Drawing for the job (mm, zero at the part's lowest x, y, z). Round coordinates to 2 decimals unless told otherwise and drop trailing zeros. Write each loop counter-clockwise with the first axis right and the second up, starting at its lowest first coordinate (ties: lowest second). Pieces come first, ordered by that corner, then holes. Notation, with made-up numbers: M -16,-29.75 L 10,-29.75 A25 ccw 10,-0.75 Z; hole C 20,42 d8. An arc over 180 degrees is marked long. Use a Markdown table: item, result. Add a question column.
1) Slice it at A-A on z = 27.5. Write the cut outline in (x, y).
2) Wall check: probe 1 along Z at (x, y) = (66.04, 2.55); probe 2 along Z at (x, y) = (61.5, 1.55); probe 3 along X at (y, z) = (1.4, 19). Give the ranges that are in metal, low to high.
3) Slice it at D-D on x = 66.04. Write the cut outline in (y, z).
4) Drop flat-ended pins along their axis: P1, Ø1.1, axis at y = 2, z = 50, coming from the -X side; P2, Ø1.1, axis at y = 3, z = 8.5, coming from the +X side; P3, Ø0.8, axis at x = 106, y = 1, coming from the -Z side. Give the stop position or say it passes through.
5) Slice it at C-C on x = 54. Write the cut outline in (y, z).
6) Slice it at B-B on y = 2.95. Give the number of separate pieces and of enclosed holes in the cut face, plus the area to 3 significant figures.
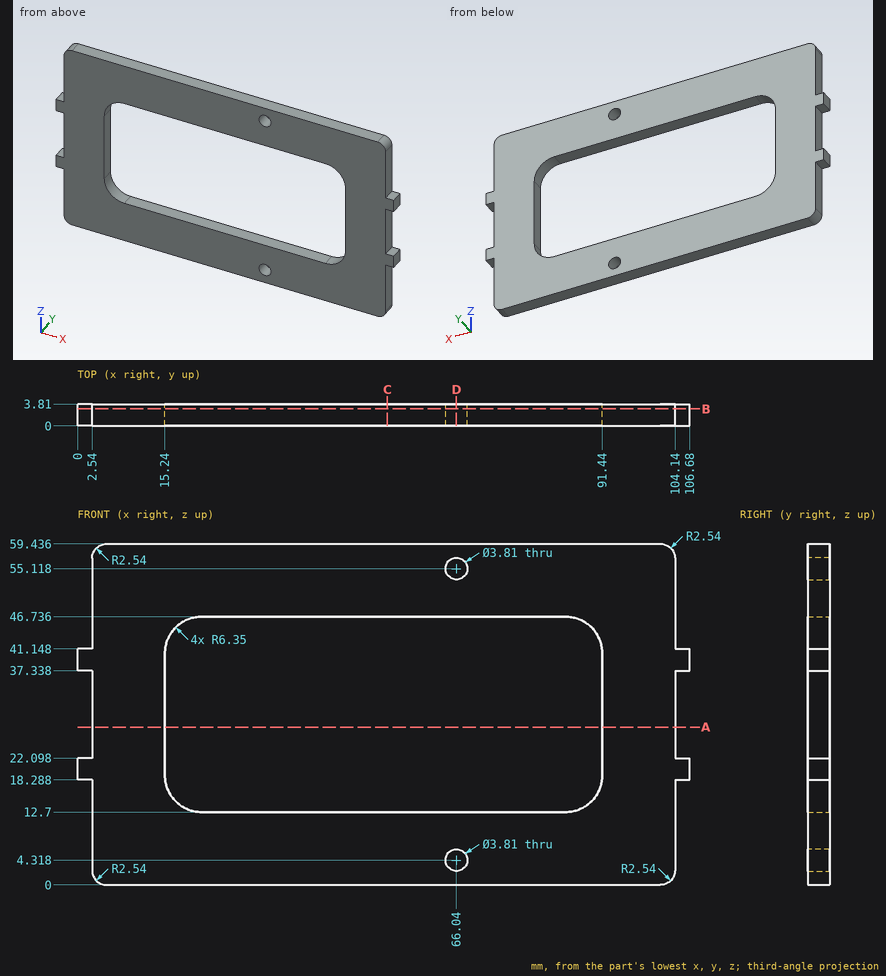
Entries:
| question | item | result |
|---|---|---|
| 1 | outline | M 2.54,0 L 15.24,0 L 15.24,3.81 L 2.54,3.81 Z; M 91.44,0 L 104.14,0 L 104.14,3.81 L 91.44,3.81 Z |
| 2 | probe 1 | z = 0 to 2.41, 6.22 to 12.7, 46.74 to 53.21, 57.02 to 59.44 |
| 2 | probe 2 | z = 0 to 12.7, 46.74 to 59.44 |
| 2 | probe 3 | x = 0 to 15.24, 91.44 to 106.68 |
| 3 | outline | M 0,0 L 3.81,0 L 3.81,2.41 L 0,2.41 Z; M 0,6.22 L 3.81,6.22 L 3.81,12.7 L 0,12.7 Z; M 0,46.74 L 3.81,46.74 L 3.81,53.21 L 0,53.21 Z; M 0,57.02 L 3.81,57.02 L 3.81,59.44 L 0,59.44 Z |
| 4 | P1 | stops at x = 2.54 |
| 4 | P2 | stops at x = 104.14 |
| 4 | P3 | stops at z = 18.29 |
| 5 | outline | M 0,0 L 3.81,0 L 3.81,12.7 L 0,12.7 Z; M 0,46.74 L 3.81,46.74 L 3.81,59.44 L 0,59.44 Z |
| 6 | separate pieces | 1 |
| 6 | enclosed holes | 3 |
| 6 | area | 3,490 mm^2 |
